Verification items for the finished model (mm, model axes). Coordinates: 2 decimals unless noted, no trailing zeros. Order: outer loops, then holes, each group sorted by start corner. A loop starts at its lowest first (then second) coordinate and runs counter-clockwise, first axis right, second up. Notation, with made-up numbers: (-4, -35.5) -> (34, -35.5) arc R28 cw to (34, 0.5) -> close; hole circle Ø2 at (-2.75, 31). An arc over 180 degrees is marked (long way). Write each question's results on one line, items separated by ' | '. Start each with the question number.
(1) Cross-section at D-D on x = 0. Enter the section's corners in (y, z), and give its area (3 significant figures).
(2) Cross-section at A-A on z = -10. Enter the section's corners in (x, y), and give its area (3 significant figures).
(3) Draft check along Z on faces 1 (the flat face through (0, 2, -20)), 2 (the flat face through (-25, 2, 0)), 3 (the cylindrical face through (21.55, 3.03, 10.73)). Enter one of: +Z half, -Z half, draft (parallel to the pull), parting line (faces both ways), or undercut.
(4) Cross-section at B-B on x = -22.5. Enter the section's corners in (y, z), and give its area (3 significant figures).
(5) Thickness scan on probe 1 along X at (y, z) = (1.6, 10); probe 2 along Z at (x, y) = (-22.5, 3.5); probe 3 along X at (y, z) = (1.25, 10.5). Record the ranges inside material, lowest first. Write a range as [from, to].
(6) Go/stop test with a flat-tipped pin: pin 1 (4 mm diameter, centred on x = 22.5, z = 10, fed in from -Y). Record where the tip stops, or that it passes through.
(7) Cross-section at C-C on y = 3.15. Enter the section's corners in (x, z), and give its area (3 significant figures).
```python
from build123d import *

# Parameters (mm, degrees)
SKETCH1_W                                           = 50
SKETCH1_H                                           = 40
SKETCH1_R                                           = 5
BOSS_EXTRUDE1_DEPTH                                 = 5
CSK_FOR_M2_COUNTERSUNK_FLAT_HEAD_SCREW1_D           = 2.4
CSK_FOR_M2_COUNTERSUNK_FLAT_HEAD_SCREW1_CSINK_D     = 4.4
CSK_FOR_M2_COUNTERSUNK_FLAT_HEAD_SCREW1_CSINK_ANGLE = 90


with BuildPart() as part:
    # Sketch1 → Boss-Extrude1 (new body)
    with BuildSketch(Plane(origin=(0, 0, 0), x_dir=(1, 0, 0), z_dir=(0, 1, 0))):
        Rectangle(SKETCH1_W, SKETCH1_H)
        with Locations(Location((0, 0, 0), (0, 0, 270))):
            Circle(SKETCH1_R, mode=Mode.SUBTRACT)
    extrude(amount=BOSS_EXTRUDE1_DEPTH)

    # CSK for M2 Countersunk Flat Head Screw1 (through all)
    with Locations(Plane(origin=(0, 0, 0), x_dir=(-1, 0, 0), z_dir=(0, -1, 0))):
        with Locations((22.5, -10), (22.5, 10), (-22.5, 10), (-22.5, -10)):
            CounterSinkHole(CSK_FOR_M2_COUNTERSUNK_FLAT_HEAD_SCREW1_D / 2, CSK_FOR_M2_COUNTERSUNK_FLAT_HEAD_SCREW1_CSINK_D / 2, counter_sink_angle=CSK_FOR_M2_COUNTERSUNK_FLAT_HEAD_SCREW1_CSINK_ANGLE)


solid = part.part
```
Results are:
1) outline: (0, -20) -> (5, -20) -> (5, -5) -> (0, -5) -> close; (0, 5) -> (5, 5) -> (5, 20) -> (0, 20) -> close | area: 150 mm2
2) outline: (-25, 0) -> (-24.7, 0) -> (-23.7, 1) -> (-23.7, 5) -> (-25, 5) -> close; (-21.3, 1) -> (-20.3, 0) -> (20.3, 0) -> (21.3, 1) -> (21.3, 5) -> (-21.3, 5) -> close; (23.7, 1) -> (24.7, 0) -> (25, 0) -> (25, 5) -> (23.7, 5) -> close | area: 224 mm2
3) face 1: -Z half | face 2: draft | face 3: undercut
4) outline: (0, -20) -> (5, -20) -> (5, -11.2) -> (1, -11.2) -> (0, -12.2) -> close; (0, -7.8) -> (1, -8.8) -> (5, -8.8) -> (5, 8.8) -> (1, 8.8) -> (0, 7.8) -> close; (0, 12.2) -> (1, 11.2) -> (5, 11.2) -> (5, 20) -> (0, 20) -> close | area: 174 mm2
5) probe 1: x = [-25, -23.7], [-21.3, 21.3], [23.7, 25] | probe 2: z = [-20, -11.2], [-8.8, 8.8], [11.2, 20] | probe 3: x = [-25, -23.59], [-21.41, 21.41], [23.59, 25]
6) pin 1: stops at y = 0.2
7) outline: (-25, -20) -> (25, -20) -> (25, 20) -> (-25, 20) -> close; hole circle Ø2.4 at (-22.5, -10); hole circle Ø2.4 at (-22.5, 10); hole circle Ø10 at (0, 0); hole circle Ø2.4 at (22.5, -10); hole circle Ø2.4 at (22.5, 10) | area: 1,900 mm2
